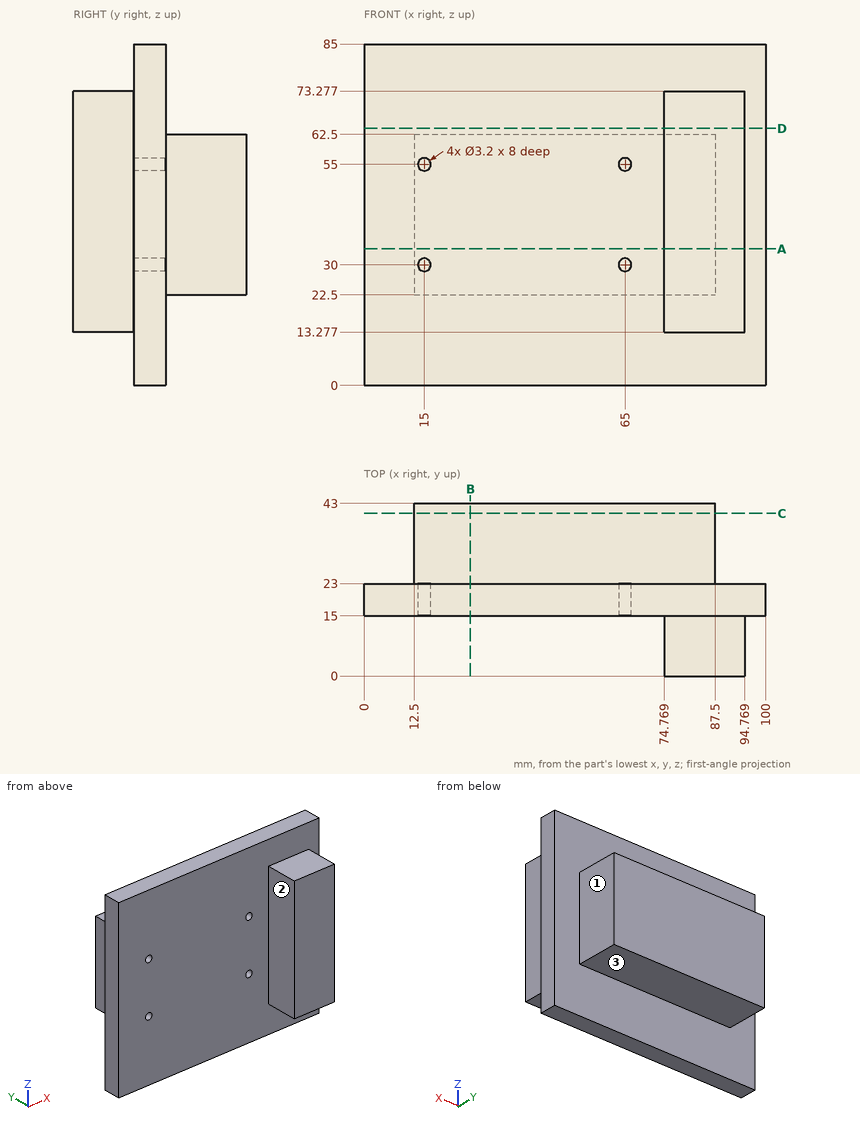
Geometry: see drawing. Coordinates: mm, zero at the bounding-box minimum. A direction names the side the tool comes from. Round coordinates to 2 decimals unless told otherwise and drop trailing zeros. Loops run counter-clockwise (first coordinate to the right, second up) from the corner with the lowest first, then second, coordinate; pieces in that order, holes last. Notation, with made-up numbers: M 81,-19 L 127,-19 A34 cw 127,14 Z; hole C 67,76.5 d9. An arc over 180 degrees is marked long. Use a Markdown table: item, result. Add a question column.
1. Section query A-A on z = 34. Return the cut outline in (x, y).
2. Reachability of the marked faces 1, 2 and 3 from +Z, -Z, +X, -X, +Y, -Y: full face, straight path, thin tool, end or side. Return the list, or none.
3. Section query D-D on z = 64. Return the cut outline in (x, y).
4. Section query B-B on x = 26.5. Return the cut outline in (y, z), then the cut area to 3 significant figures.
5. Line query: line 1 (Z direction, x = 65, y = 17); line 2 (Y direction, x = 59.5, z = 16); line 3 (Z direction, x = 35, y = 33). Output: solid intervals per line, ascending.
6. Contact query for flat-ended pins moving along their axis: P1, Ø3, axis at x = 20.5, z = 75.5, coming from the +Y side; P2, Ø10, axis at x = 17, z = 73, coming from the -Y side; P3, Ø1.6, axis at x = 15, z = 55, coming from the -Y side. Output: stop coordinate, or through.
7. Section query C-C on y = 40.5. Return the cut outline in (x, z), then the cut area to 3 significant figures.
Reported:
| question | item | result |
|---|---|---|
| 1 | outline | M 0,15 L 74.77,15 L 74.77,0 L 94.77,0 L 94.77,15 L 100,15 L 100,23 L 87.5,23 L 87.5,43 L 12.5,43 L 12.5,23 L 0,23 Z |
| 2 | face 1 | +Z, -Z, +X, +Y |
| 2 | face 2 | +Z, -Z, -X, -Y |
| 2 | face 3 | -Z, +X, -X, +Y |
| 3 | outline | M 0,15 L 74.77,15 L 74.77,0 L 94.77,0 L 94.77,15 L 100,15 L 100,23 L 0,23 Z |
| 4 | outline | M 15,0 L 23,0 L 23,22.5 L 43,22.5 L 43,62.5 L 23,62.5 L 23,85 L 15,85 Z |
| 4 | area | 1,480 mm² |
| 5 | line 1 | z = 0 to 28.4, 31.6 to 53.4, 56.6 to 85 |
| 5 | line 2 | y = 15 to 23 |
| 5 | line 3 | z = 22.5 to 62.5 |
| 6 | P1 | stops at y = 23 |
| 6 | P2 | stops at y = 15 |
| 6 | P3 | stops at y = 23 |
| 7 | outline | M 12.5,22.5 L 87.5,22.5 L 87.5,62.5 L 12.5,62.5 Z |
| 7 | area | 3,000 mm² |
